from build123d import *

# Parameters (mm, degrees)
ESQUISSE1_R             = 25
ESQUISSE1_R_2           = 19
ESQUISSE3_R             = 27.5
ESQUISSE3_R_2           = 23.5
ENL_V_MAT_EXTRU_1_DEPTH = 30
ESQUISSE4_R             = 27.5
ESQUISSE4_R_2           = 23.5
ENL_V_MAT_EXTRU_2_DEPTH = 30


with BuildPart() as part:
    # Balayage1: sweep along a path in Esquisse2
    with BuildLine(Plane(origin=(0, 0, 0), x_dir=(0, 0, -1), z_dir=(1, 0, 0))) as balayage1_path:
        Line((0, 0), (31.347693674, 0))
        ThreePointArc((31.347693674, 0), (48.252424143, 3.747688519), (61.989471399, 14.288495613))
        Line((61.989471399, 14.288495613), (82.139380484, 38.302222156))
    # Esquisse1 → Balayage1 (sweep)
    with BuildSketch(Plane.XY):
        Circle(ESQUISSE1_R)
        Circle(ESQUISSE1_R_2, mode=Mode.SUBTRACT)
    sweep(path=balayage1_path.line)

    # Esquisse3 → Enlèv. mat.-Extru.1 (cut)
    with BuildSketch(Plane.XY):
        Circle(ESQUISSE3_R)
        Circle(ESQUISSE3_R_2, mode=Mode.SUBTRACT)
    extrude(amount=-ENL_V_MAT_EXTRU_1_DEPTH, mode=Mode.SUBTRACT)

    # Esquisse4 → Enlèv. mat.-Extru.2 (cut)
    with BuildSketch(Plane(origin=(0, 62.922415981, -52.798176043), x_dir=(1, 0, 0), z_dir=(0, 0.7660444431189795, -0.6427876096865377))):
        with Locations((0, 38.302222156)):
            Circle(ESQUISSE4_R)
        with Locations(Location((0, 38.302222156, 0), (0, 0, 270))):
            Circle(ESQUISSE4_R_2, mode=Mode.SUBTRACT)
    extrude(amount=-ENL_V_MAT_EXTRU_2_DEPTH, mode=Mode.SUBTRACT)


solid = part.part
Could you check a few things on this model? Use its own coordinates, in mm. A direction names the side the tool comes from. Give positions to 0.01 mm unless a question says otherwise; leave off trailing zeros. Order: outer loops, then holes, each group sorted by start corner. A loop starts at its lowest first (then second) coordinate and runs counter-clockwise, first axis right, second up. Notation, with made-up numbers: (2.25, 18.5) -> (38.25, 18.5) arc R25 ccw to (38.25, 55.5) -> close; hole circle Ø2 at (30, 88.5). An arc over 180 degrees is marked (long way). Return JSON: item names as keys, results as strings.
1. Thinking about a two-plate mould opening in Y: for faces 3 (the cylindrical face through (23.846, 9.985, -68.181)), 4 (the flat face through (-17.3, 32.78, -88.72)), 5 (the flat face through (22.11, 21.2, -55.85)), which applies, pulls with the +Y half, pulls with the -Y half, needs draft (parallel to the pull), parting line crosses it, or undercut?
Answer list:
{"face 3": "parting line crosses it", "face 4": "pulls with the +Y half", "face 5": "undercut"}
2. Imagine slicing it at A-A on x = 0. List the corners of the cut face in (y, z) for me, then the cut area to 3 significant figures.
Answer list:
{"outline": "(-25, -31.35) arc R65 ccw to (-1.78, -81.14) -> (-0.75, -82.01) -> (0.22, -80.86) -> (23.2, -100.14) -> (26.09, -96.69) -> (2.08, -76.54) arc R59 cw to (-19, -31.35) -> (-19, 0) -> (-23.5, 0) -> (-23.5, -30) -> (-25, -30) -> close; (19, -31.35) arc R21 ccw to (26.5, -47.43) -> (50.52, -67.58) -> (53.41, -64.14) -> (30.43, -44.85) -> (31.39, -43.7) -> (30.36, -42.84) arc R15 cw to (25, -31.35) -> (25, -30) -> (23.5, -30) -> (23.5, 0) -> (19, 0) -> close", "area": "991 mm2"}
3. Imagine slicing it at C-C on x = -13. List the corners of the cut face in (y, z) for me, then the cut area to 3 significant figures.
Answer list:
{"outline": "(-21.35, -31.35) arc R61.35 ccw to (0.56, -78.35) -> (1.59, -79.21) -> (2.74, -77.85) -> (25.72, -97.14) -> (29.4, -92.75) -> (5.38, -72.6) arc R53.86 cw to (-13.86, -31.35) -> (-13.86, 0) -> (-19.58, 0) -> (-19.58, -30) -> (-21.35, -30) -> close; (13.86, -31.35) arc R26.14 ccw to (23.2, -51.37) -> (47.21, -71.52) -> (50.89, -67.14) -> (27.9, -47.86) -> (29.05, -46.5) -> (28.01, -45.63) arc R18.65 cw to (21.35, -31.35) -> (21.35, -30) -> (19.58, -30) -> (19.58, 0) -> (13.86, 0) -> close", "area": "1,250 mm2"}
4. For pin 1 Ø10 at (x, y) = (3.5, -0.5) entering from +Z; pin 2 Ø10 at (x, z) = (-4.5, -16.5) entering from +Y; pin 3 Ø1.5 at (x, z) = (-2.5, -79.5) entering from +Y; pin 4 Ø15 at (x, y) = (0, 12.5) entering from +Z, each with a flat end and sliding along its axis, tell me the tip position at first contact or that it passes through.
Answer list:
{"pin 1": "stops at z = -68.13", "pin 2": "stops at y = 23.5", "pin 3": "stops at y = 6.76", "pin 4": "stops at z = 0"}
5. I need wall thicknesses on line 1 (Y direction, x = 0, z = -14); line 2 (Y direction, x = -6, z = -5.5); line 3 (X direction, y = 22.5, z = -65). Which ranges of each line are inside material? Lowest first, please. Write a range as from..to.
Answer list:
{"line 1": "y = -23.5..-19, 19..23.5", "line 2": "y = -22.72..-18.03, 18.03..22.72", "line 3": "x = -23.31..-18.77, 18.77..23.31"}
6. Imagine slicing it at B-B on z = -25.5. List the corners of the cut face in (x, y) for me, then the cut area to 3 significant figures.
Answer list:
{"outline": "circle Ø47 at (0, 0); hole circle Ø38 at (0, 0)", "area": "601 mm2"}
7. On a 3-axis mill with a long thin cutter (end or side, diameter ignored), from which of +Z, -Z, +X, -X, +Y, -Y can I reach the whole of each face in a straight line? I mean faces 1 (the cylindrical face through (8.767, 16.856, -15.893)), 2 (the flat face through (9, -17, 0)). Say none if no direction works.
Answer list:
{"face 1": "+Z", "face 2": "+Z, +X, -X, +Y, -Y"}
